from build123d import *

# Parameters (mm, degrees)
REVOLVE1_ANGLE = 180


with BuildPart() as part:
    # Sketch3 → Revolve1 (revolve, symmetric)
    with BuildSketch(Plane(origin=(0, 0, 0), x_dir=(0, 0, -1), z_dir=(1, 0, 0))) as revolve1_sk:
        Polygon((-100, -22.15), (-25, -50), (25, -50), (55.161579892, -36), (70.161579892, -36), (100, -22.15), (100, -19.945050391), (69.720036749, -34), (54.720036749, -34), (24.558456857, -48), (-24.640654181, -48), (-100, -20.016562919), align=None)
    revolve(axis=Axis((0, 0, 100), (0, 0, -1)), revolution_arc=REVOLVE1_ANGLE / 2)
    revolve(revolve1_sk.sketch, axis=Axis((0, 0, 100), (0, 0, 1)), revolution_arc=REVOLVE1_ANGLE / 2)


solid = part.part
Could you check a few things on this model? Use its own coordinates, in mm. A direction names the side the tool comes from. Round coordinates to 2 decimals unless told otherwise and drop trailing zeros. Write each loop counter-clockwise with the first axis right and the second up, starting at its lowest first coordinate (ties: lowest second). Pieces come first, ordered by that corner, then holes. Notation, with made-up numbers: (-14.75, 77) - (41.25, 77) arc R18 cw to (41.25, 81) - close; hole circle Ø3 at (63, 70). An arc over 180 degrees is marked (long way). Use a Markdown table: item, result.
Q1. Thinking about a two-plate mould opening in X: for faces 1 (the flat face through (-48.3, 0, 0.5)), 2 (the cylindrical face through (-0.75, -33.99, -62.12)), 3 (the cylindrical face through (-0.79, -35.99, -62.77)), which applies, released by +X, released by -X, zero draft, split by the parting line, or undercut?
Output values:
| item | result |
|---|---|
| face 1 | zero draft |
| face 2 | undercut |
| face 3 | split by the parting line |
Q2. I want a section at B-B (z = 5.5). List the corners of the cut face in (x, y) for me.
Output values:
| item | result |
|---|---|
| outline | (-50, 0) arc R50 ccw to (50, 0) - (48, 0) arc R48 cw to (-48, 0) - close |
Q3. I want a section at C-C (z = 65). List the corners of the cut face in (x, y) for me, plus the area to 3 significant figures.
Output values:
| item | result |
|---|---|
| outline | (-35.15, 0) arc R35.15 ccw to (35.15, 0) - (33.01, 0) arc R33.01 cw to (-33.01, 0) - close |
| area | 228 mm2 |
Q4. For pin 1 (10 mm diameter, centred on x = 2, z = -33, fed in from +Y); pin 2 (10 mm diameter, centred on x = 28.5, y = -19, fed in from -Z); pin 3 (1.5 mm diameter, centred on y = -26, z = -15, fed in from -X), each with a flat end and sliding along its axis, tell me the tip position at first contact or that it passes through.
Output values:
| item | result |
|---|---|
| pin 1 | y = -41.7 |
| pin 2 | z = -84.7 |
| pin 3 | x = -43.16 |
Q5. I want a section at A-A (x = 0). List the corners of the cut face in (y, z) for me, plus the area to 3 significant figures.
Output values:
| item | result |
|---|---|
| outline | (-50, -25) - (-36, -55.16) - (-36, -70.16) - (-22.15, -100) - (-19.95, -100) - (-34, -69.72) - (-34, -54.72) - (-48, -24.56) - (-48, 24.64) - (-20.02, 100) - (-22.15, 100) - (-50, 25) - close |
| area | 422 mm2 |
Q6. Please list where these lines run through material, in increasing order: L1, parallel to Z at x = -13.5, y = -30.5; L2, parallel to X at y = -32, z = 35; L3, parallel to X at y = -24, z = -23.5.
Output values:
| item | result |
|---|---|
| L1 | -75.86 to -71.11, 64.08 to 69.83 |
| L2 | -33.44 to -30.42, 30.42 to 33.44 |
| L3 | -43.86 to -41.57, 41.57 to 43.86 |
Q7. For faces 4 (the conical face through (-0.6, -27.43, -88.61)), 5 (the conical face through (-0.84, -37.98, -46.13)), which set-ups out of +Z, -Z, +X, -X, +Y, -Y let a thin tool reach every point of the face, with its end or its side?
Output values:
| item | result |
|---|---|
| face 4 | -Z, -Y |
| face 5 | +Y |
